from build123d import *

# Parameters (mm, degrees)
SKETCH1_W                      = 20.2
SKETCH1_H                      = 18
BOSS_EXTRUDE1_DEPTH            = 5.75
M2_CLEARANCE_HOLE1_D           = 2.4
M2_CLEARANCE_HOLE1_CSINK_D     = 2.45
M2_CLEARANCE_HOLE1_CSINK_ANGLE = 90
SKETCH5_W                      = 5.8
SKETCH5_H                      = 8
BOSS_EXTRUDE2_DEPTH            = 60
SKETCH6_R                      = 4.0625
CUT_EXTRUDE1_DEPTH             = 5.75
SKETCH7_R                      = 3.25
CUT_EXTRUDE2_DEPTH             = 5.75
FILLET1_R                      = 2
M2_CLEARANCE_HOLE2_D           = 2.4
M2_CLEARANCE_HOLE2_DEPTH       = 5.75
M2_CLEARANCE_HOLE2_TIP         = 0.721032743
SKETCH11_W                     = 5
SKETCH11_H                     = 8
SKETCH11_W_2                   = 7
SKETCH11_H_2                   = 4
BOSS_EXTRUDE3_DEPTH            = 5.75
SKETCH12_W                     = 5
SKETCH12_H                     = 8
SKETCH12_W_2                   = 7
SKETCH12_H_2                   = 4
BOSS_EXTRUDE4_DEPTH            = 5.75
FILLET2_R                      = 2
SKETCH14_W                     = 24.4
SKETCH14_H                     = 1
CUT_EXTRUDE3_DEPTH             = 2
FILLET3_R                      = 1
FILLET4_R                      = 1


with BuildPart() as part:
    # Sketch1 → Boss-Extrude1 (new body)
    with BuildSketch(Plane(origin=(0, 0, 0), x_dir=(1, 0, 0), z_dir=(0, 1, 0))):
        with Locations((1, 0)):
            Rectangle(SKETCH1_W, SKETCH1_H)
    boss_extrude1 = extrude(amount=BOSS_EXTRUDE1_DEPTH)

    # M2 Clearance Hole1 (through all)
    with Locations(Plane(origin=(0, 5.75, 0), x_dir=(1, 0, 0), z_dir=(0, 1, 0))):
        with Locations((-6.1, 6), (5.9, 6), (-6.1, -6), (5.9, -6)):
            CounterSinkHole(M2_CLEARANCE_HOLE1_D / 2, M2_CLEARANCE_HOLE1_CSINK_D / 2, counter_sink_angle=M2_CLEARANCE_HOLE1_CSINK_ANGLE)

    # Sketch5 → Boss-Extrude2 (add)
    with BuildSketch(Plane(origin=(0, 5.75, 0), x_dir=(1, 0, 0), z_dir=(0, 1, 0))):
        with Locations((-11.2, 0.5)):
            Rectangle(SKETCH5_W, SKETCH5_H)
        Polygon((3.5, -7.6), (-1.5, -7.6), (-3.5, -7.6), (-3.5, -9), (-3.5, -13), (3.5, -13), (3.5, -9), align=None)
        with Locations((13.2, 0.5)):
            Rectangle(SKETCH5_W, SKETCH5_H)
    extrude(amount=BOSS_EXTRUDE2_DEPTH)

    # Sketch6 → Cut-Extrude1 (cut)
    with BuildSketch(Plane(origin=(0, 5.75, 0), x_dir=(1, 0, 0), z_dir=(0, 1, 0))):
        with Locations(Location((0, 0, 0), (0, 0, 270))):
            Circle(SKETCH6_R)
    extrude(amount=-CUT_EXTRUDE1_DEPTH, mode=Mode.SUBTRACT)

    # Mirror1: Boss-Extrude1 across plane
    add(boss_extrude1.mirror(Plane.ZX.offset(35.75)))

    # Sketch7 → Cut-Extrude2 (cut)
    with BuildSketch(Plane(origin=(0, 71.5, 0), x_dir=(1, 0, 0), z_dir=(0, 1, 0))):
        with Locations(Location((0, 0, 0), (0, 0, 270))):
            Circle(SKETCH7_R)
    extrude(amount=-CUT_EXTRUDE2_DEPTH, mode=Mode.SUBTRACT)

    # Fillet1
    fillet1_edges = [part.edges().sort_by_distance(p)[0] for p in [
        (11.1, 68.625, -9),
        (11.1, 68.625, 9),
        (-9.1, 68.625, 9),
        (-9.1, 68.625, -9),
        (11.1, 2.875, 9),
        (-9.1, 2.875, 9),
        (-9.1, 2.875, -9),
        (11.1, 2.875, -9),
    ]]
    fillet(fillet1_edges, radius=FILLET1_R)

    # M2 Clearance Hole2
    with Locations(Plane(origin=(0, 71.5, 0), x_dir=(1, 0, 0), z_dir=(0, 1, 0))):
        with Locations((-4.142372511, -2.800133921), (4.142372511, 2.800133921)):
            Hole(M2_CLEARANCE_HOLE2_D / 2, depth=M2_CLEARANCE_HOLE2_DEPTH)
            with Locations((0, 0, -(M2_CLEARANCE_HOLE2_DEPTH + M2_CLEARANCE_HOLE2_TIP / 2))):  # 118° drill point
                Cone(0, M2_CLEARANCE_HOLE2_D / 2, M2_CLEARANCE_HOLE2_TIP, mode=Mode.SUBTRACT)

    # Sketch11 → Boss-Extrude3 (add)
    with BuildSketch(Plane(origin=(0, 65.75, 0), x_dir=(1, 0, 0), z_dir=(0, 1, 0))):
        with Locations((-11.6, 0.5)):
            Rectangle(SKETCH11_W, SKETCH11_H)
        with Locations((13.6, 0.5)):
            Rectangle(SKETCH11_W, SKETCH11_H)
        with Locations((0, -11)):
            Rectangle(SKETCH11_W_2, SKETCH11_H_2)
    extrude(amount=BOSS_EXTRUDE3_DEPTH)

    # Sketch12 → Boss-Extrude4 (add)
    with BuildSketch(Plane.XZ.offset(-5.75)):
        with Locations((-11.6, -0.5)):
            Rectangle(SKETCH12_W, SKETCH12_H)
        with Locations((0, 11)):
            Rectangle(SKETCH12_W_2, SKETCH12_H_2)
        with Locations((13.6, -0.5)):
            Rectangle(SKETCH12_W, SKETCH12_H)
    extrude(amount=BOSS_EXTRUDE4_DEPTH)

    # Fillet2
    fillet2_edges = [part.edges().sort_by_distance(p)[0] for p in [
        (-14.1, 35.75, -4.5),
        (-14.1, 35.75, 3.5),
        (3.5, 35.75, 13),
        (-3.5, 35.75, 13),
        (10.3, 35.75, 3.5),
        (10.3, 35.75, -4.5),
    ]]
    fillet(fillet2_edges, radius=FILLET2_R)

    # Sketch14 → Cut-Extrude3 (cut)
    with BuildSketch(Plane(origin=(0, 0, -4.5), x_dir=(-1, 0, 0), z_dir=(0, 0, -1))):
        with Locations((-0.1, 10.5)):
            Rectangle(SKETCH14_W, SKETCH14_H)
    extrude(amount=-CUT_EXTRUDE3_DEPTH, mode=Mode.SUBTRACT)

    # Fillet3
    fillet3_edges = [part.edges().sort_by_distance(p)[0] for p in [
        (10.885786438, 10, -3.914213562),
        (10.885786438, 11, -3.914213562),
        (-10.2, 10, -4.5),
        (-10.2, 11, -4.5),
    ]]
    fillet(fillet3_edges, radius=FILLET3_R)

    # Fillet4
    fillet4_edges = [part.edges().sort_by_distance(p)[0] for p in [
        (-8.3, 11, -3),
        (-8.3, 11.292893219, -4.207106781),
        (-8.3, 10, -3),
        (-8.3, 9.707106781, -4.207106781),
        (16.1, 35.75, -4.5),
        (-8.3, 38.875, -4.5),
        (-8.3, 7.375, -4.5),
    ]]
    fillet(fillet4_edges, radius=FILLET4_R)


solid = part.part
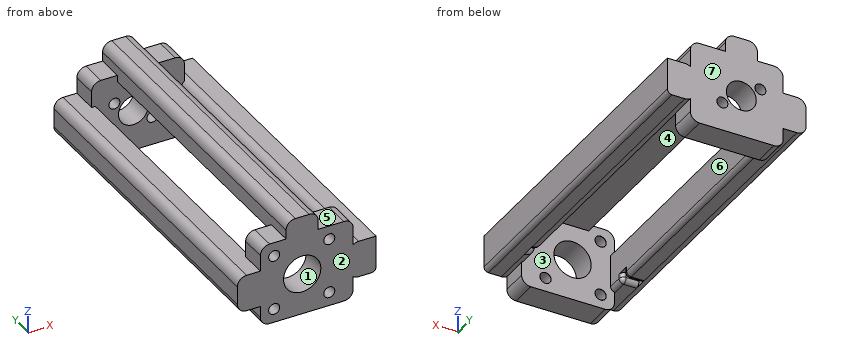
Can you work these out from the model? Positions are in its coordinate system, mm. Face numbers are marked on the shaded views. A direction names the side the tool comes from. Round coordinates to 2 decimals unless told otherwise and drop trailing zeros. Loops run counter-clockwise (first coordinate to the right, second up) from the corner with the lowest first, then second, coordinate; pieces in that order, holes last. Notation, with made-up numbers: (39, 7.5) - (48, 7.5) arc R15 ccw to (48, 36.5) - close; hole circle Ø4 at (-10.5, 25.5). An arc over 180 degrees is marked (long way). Answer in a Markdown table with one row per item. Add a question column.
Q1. I want a section at A-A on z = -6. List the corners of the cut face in (x, y) for me (3 decimals), and give its area (3 significant figures).
Q2. I need wall thicknesses on L1, parallel to Z at x = -6.1, y = 3.25; L2, parallel to X at y = 3.4, z = -6; L3, parallel to Y at x = -12, z = -2.75. Which ranges of each line are inside material? Lowest first, please.
Q3. For pin 1 Ø5 at (x, y) = (-4.5, 38.5) entering from -Z; pin 2 Ø2 at (x, y) = (-3.5, 51.5) entering from +Z; pin 3 Ø1 at (y, z) = (41, 10) entering from -X, each with a flat end and sliding along its axis, tell me the tip position at first contact or that it passes through.
Q4. I want a section at D-D on z = 0. List the corners of the cut face in (x, y) for me, and give its area (3 significant figures).
Q5. Which directions (+Z, -Z, +X, -X, +Y, -Y) give clear straight access to the entire face, cutting with the end or side of a thin tool? Please do the marked faces 4, 5, 6 and 7.
Q6. We'd pull the mould along Y, two halves only. Please class the marked faces 1, 2 and 3: pulls with the +Y half, pulls with the -Y half, needs draft (parallel to the pull), parting line crosses it, or undercut.
Q7. I want a section at B-B on y = 26.5. List the corners of the cut face in (x, z) for me, and give its area (3 significant figures).
Q8. I want a section at C-C on x = -6.1. List the corners of the cut face in (y, z) for me (3 decimals), and give its area (3 significant figures).
A:
| question | item | result |
|---|---|---|
| 1 | outline | (-9.1, 0) - (-7.3, 0) - (-7.3, 5.725) - (-7.325, 5.75) - (-9.1, 5.75) - close; (-9.1, 65.75) - (11.1, 65.75) - (11.1, 71.5) - (-9.1, 71.5) - close; (-4.9, 0) - (4.7, 0) - (4.7, 5.725) - (4.675, 5.75) - (-4.875, 5.75) - (-4.9, 5.725) - close; (7.1, 0) - (11.1, 0) - (11.1, 5.75) - (7.125, 5.75) - (7.1, 5.725) - close |
| 1 | area | 205 mm^2 |
| 2 | L1 | -9 to -7.2, -4.8 to 4.8, 7.2 to 9 |
| 2 | L2 | -9.1 to -7.3, -4.9 to 4.7, 7.1 to 11.1 |
| 2 | L3 | 0 to 10, 11 to 71.5 |
| 3 | pin 1 | z = 7.6 |
| 3 | pin 2 | z = 12.73 |
| 3 | pin 3 | x = -3.5 |
| 4 | outline | (-14.1, 0) - (-4.06, 0) - (-4.06, 5.75) - (-8.3, 5.75) - (-8.3, 65.75) - (-3.25, 65.75) - (-3.25, 71.5) - (-14.1, 71.5) - close; (3.25, 65.75) - (10.3, 65.75) - (10.3, 5.75) - (4.06, 5.75) - (4.06, 0) - (16.1, 0) - (16.1, 71.5) - (3.25, 71.5) - close |
| 4 | area | 959 mm^2 |
| 5 | face 4 | -Z, +X, -X |
| 5 | face 5 | +Z, +X, +Y, -Y |
| 5 | face 6 | +Z, -Z |
| 5 | face 7 | +Z, -Z, +X, -X, +Y |
| 6 | face 1 | needs draft |
| 6 | face 2 | pulls with the -Y half |
| 6 | face 3 | undercut |
| 7 | outline | (-14.1, -2.5) arc R2 ccw to (-12.1, -4.5) - (-9.3, -4.5) arc R1 ccw to (-8.3, -3.5) - (-8.3, 3.5) - (-12.1, 3.5) arc R2 ccw to (-14.1, 1.5) - close; (-3.5, 7.6) - (3.5, 7.6) - (3.5, 11) arc R2 ccw to (1.5, 13) - (-1.5, 13) arc R2 ccw to (-3.5, 11) - close; (10.3, -2.5) arc R2 ccw to (12.3, -4.5) - (15.1, -4.5) arc R1 ccw to (16.1, -3.5) - (16.1, 3.5) - (12.3, 3.5) arc R2 ccw to (10.3, 1.5) - close |
| 7 | area | 125 mm^2 |
| 8 | outline | (0, -9) - (5.75, -9) - (5.75, -7.225) - (5.725, -7.2) - (0, -7.2) - close; (0, -4.8) - (5.725, -4.8) - (5.75, -4.775) - (5.75, 4.775) - (5.725, 4.8) - (0, 4.8) - close; (0, 7.2) - (5.725, 7.2) - (5.75, 7.225) - (5.75, 9) - (0, 9) - close; (65.75, -9) - (71.5, -9) - (71.5, 9) - (65.75, 9) - close |
| 8 | area | 179 mm^2 |
